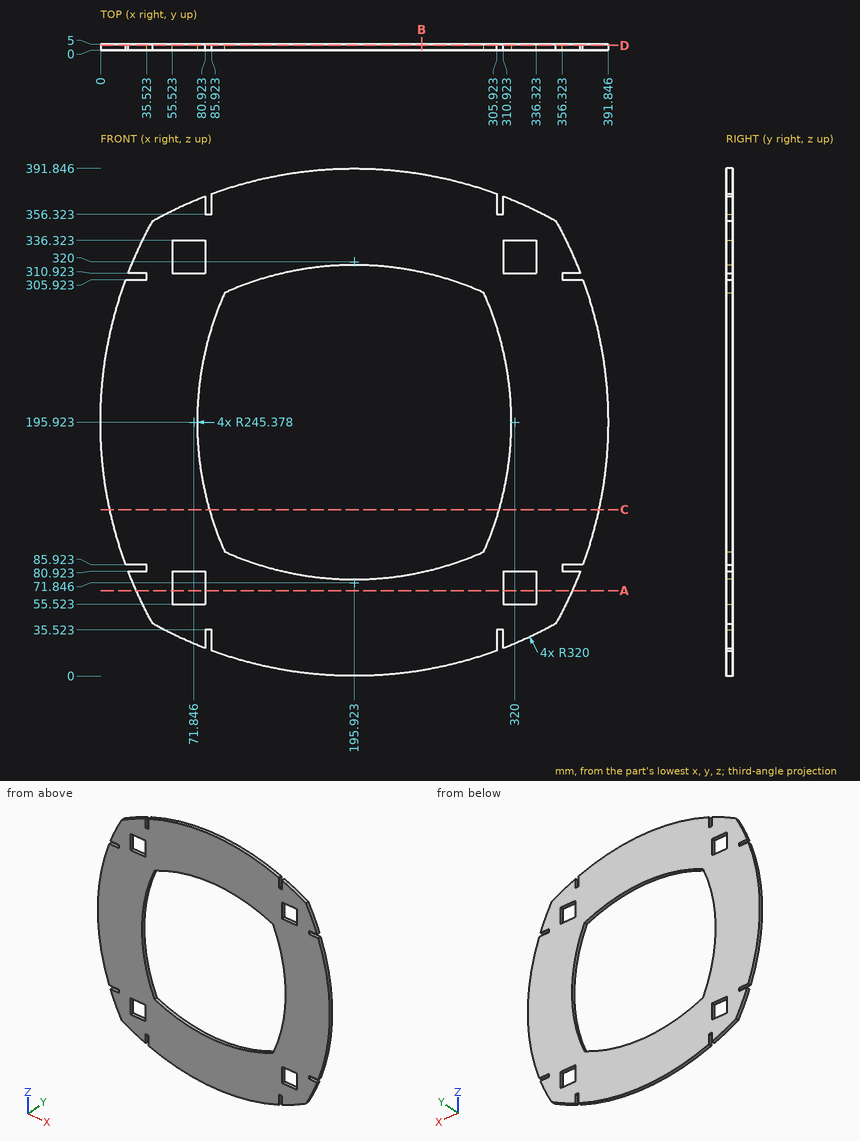
Job drawing, mm, ordinate dimensions from the low corner. One solid piece. Give positions to 0.01 mm unless a question says otherwise; leave off trailing zeros. Loops run counter-clockwise (first coordinate to the right, second up) from the corner with the lowest first, then second, coordinate; pieces in that order, holes last. Notation, with made-up numbers: (60.5, 14) - (99.5, 14) arc R33 cw to (99.5, 42) - close; hole circle Ø8 at (-10, -35). An arc over 180 degrees is marked (long way). Use one line per item in the form item = value.
(1) Cut at C-C (z = 128.5). Give the cut face in (x, y), then the cut area to 3 significant figures.
Determined:
outline = (7.18, 0) - (84.07, 0) - (84.07, 5) - (7.18, 5) - close; (307.78, 0) - (384.66, 0) - (384.66, 5) - (307.78, 5) - close
area = 769 mm^2
(2) Cut at D-D (y = 4). Count the separate pieces of the cut face and the enclosed holes in it, then the cut area to 3 significant figures.
Determined:
separate_pieces = 1
enclosed_holes = 5
area = 76,100 mm^2
(3) Drop flat-ended pins along their axis: P1, Ø1.5, axis at x = 24, y = 2.5, coming from the +Z side (1 decimal); P2, Ø2.5, axis at y = 3, z = 67, coming from the +X side; P3, Ø1.5, axis at x = 328.5, y = 1.5, coming from the +Z side; P4, Ø8, axis at x = 326.5, z = 241.5, coming from the -Y side. Give the stop position or say it passes through.
Determined:
P1 = 319.3
P2 = 365.27
P3 = 363.43
P4 = 0
(4) Drill centre lines: L1, parallel to X at y = 0.4, z = 67; L2, parallel to X at y = 0.9, z = 25.5 (1 decimal); L3, parallel to Z at x = 64, y = 2.35. Where is each one in solid material? Low to high.
Determined:
L1 = 27.12 to 55.52, 80.92 to 310.92, 336.32 to 364.73
L2 = 70.7 to 80.9, 85.9 to 305.9, 310.9 to 321.1
L3 = 28.46 to 55.52, 80.92 to 310.92, 336.32 to 363.39
(5) Cut at B-B (x = 248). Give the cut face in (y, z) (1 decimal).
Determined:
outline = (0, 4.3) - (5, 4.3) - (5, 80.2) - (0, 80.2) - close; (0, 311.6) - (5, 311.6) - (5, 387.6) - (0, 387.6) - close
(6) Cut at A-A (z = 66). Give the cut face in (x, y) (1 decimal), then the cut area to 3 significant figures.
Determined:
outline = (27.6, 0) - (55.5, 0) - (55.5, 5) - (27.6, 5) - close; (80.9, 0) - (310.9, 0) - (310.9, 5) - (80.9, 5) - close; (336.3, 0) - (364.3, 0) - (364.3, 5) - (336.3, 5) - close
area = 1,430 mm^2
